from build123d import *

# Parameters (mm, degrees)
SKETCH_1_R                   = 26.5
EXTRUDE_2_DEPTH              = 5
SKETCH_3_R                   = 15
EXTRUDE_3_DEPTH              = 13
EXTRUDE_START                = 26.5
SKETCH_4_R                   = 15
EXTRUDE_4_DEPTH              = 26.5
HOLE_WIZARD_M4_1_D           = 3.3
HOLE_WIZARD_M4_1_CSINK_D     = 4.05
HOLE_WIZARD_M4_1_CSINK_ANGLE = 90
PATTERN_CIRCULAR_1_COUNT     = 6
SKETCH_7_R                   = 7.45
CUT_EXTRUDE_1_DEPTH          = 44.5
SKETCH_8_W                   = 5.01
SKETCH_8_H                   = 5
CUT_EXTRUDE_2_DEPTH          = 44.5


with BuildPart() as part:
    # 草图1 → 凸台-拉伸2 (new body)
    with BuildSketch(Plane(origin=(0, 0, 0), x_dir=(1, 0, 0), z_dir=(0, 1, 0))):
        with Locations(Location((0, 0, 0), (0, 0, 270))):
            Circle(SKETCH_1_R)
    extrude(amount=EXTRUDE_2_DEPTH)

    # 草图3 → 凸台-拉伸3 (add)
    with BuildSketch(Plane(origin=(0, 5, 0), x_dir=(1, 0, 0), z_dir=(0, 1, 0))):
        with Locations(Location((0, 0, 0), (0, 0, 90))):
            Circle(SKETCH_3_R)
    extrude(amount=EXTRUDE_3_DEPTH)

    # 草图4 → 凸台-拉伸4 (add)
    with BuildSketch(Plane.XZ.offset(EXTRUDE_START)):
        with Locations(Location((0, 0, 0), (0, 0, 270))):
            Circle(SKETCH_4_R)
    extrude(amount=-EXTRUDE_4_DEPTH)

    # M4 螺纹孔1 (through all)
    with Locations(Plane(origin=(22, 5, 0), x_dir=(0, 0, 1), z_dir=(0, 1, 0))):
        with Locations((0, 0)):
            hole_wizard_m4_1 = CounterSinkHole(HOLE_WIZARD_M4_1_D / 2, HOLE_WIZARD_M4_1_CSINK_D / 2, counter_sink_angle=HOLE_WIZARD_M4_1_CSINK_ANGLE)

    # 阵列(圆周)1: M4 螺纹孔1 ×6 about axis
    pattern_circular_1_axis = Axis((0, 0, 0), (0, 1, 0))
    for i in range(1, PATTERN_CIRCULAR_1_COUNT):
        add(hole_wizard_m4_1.rotate(pattern_circular_1_axis, i * 360 / PATTERN_CIRCULAR_1_COUNT), mode=Mode.SUBTRACT)

    # 草图7 → 切除-拉伸1 (cut)
    with BuildSketch(Plane(origin=(0, 18, 0), x_dir=(1, 0, 0), z_dir=(0, 1, 0))):
        with Locations(Location((0, 0, 0), (0, 0, 270))):
            Circle(SKETCH_7_R)
    extrude(amount=-CUT_EXTRUDE_1_DEPTH, mode=Mode.SUBTRACT)

    # 草图8 → 切除-拉伸2 (cut)
    with BuildSketch(Plane(origin=(0, 18, 0), x_dir=(1, 0, 0), z_dir=(0, 1, 0))):
        with Locations((0, -7.5)):
            Rectangle(SKETCH_8_W, SKETCH_8_H)
    extrude(amount=-CUT_EXTRUDE_2_DEPTH, mode=Mode.SUBTRACT)


solid = part.part
The model under review builds one solid part; all positions refer to its coordinate system, in mm. A direction names the side the tool comes from. Round coordinates to 2 decimals unless told otherwise and drop trailing zeros. Order: outer loops, then holes, each group sorted by start corner. A loop starts at its lowest first (then second) coordinate and runs counter-clockwise, first axis right, second up. Notation, with made-up numbers: (39, -22.75) -> (82, -22.75) arc R25 ccw to (82, -8.75) -> close; hole circle Ø7 at (-37, 39.25). An arc over 180 degrees is marked (long way). Use CSV: the item, a comma, the result in double quotes. Start each with the question number.
(1) Tool access review of faces 1 (the face through (0.66, -13.436, 14.985)), 2 (the face through (7, -26.5, -3)), 3 (the face through (0, -4, 10)): name each direction out of +Z, -Z, +X, -X, +Y, -Y from which nothing blocks a thin tool from reaching the whole face with its end or side.
(2) Consider section B-B on x = -4. Write out the cut boundary in (y, z), and give its area (3 significant figures).
(3) Consider section A-A on z = 0. Write out the cut boundary in (x, y) (3 decimals).
(4) Consider section D-D on y = 2.5. Write out the cut boundary in (x, z) (3 decimals).
(5) Insertion check: pin 1 (6 mm diameter, centred on x = 13.5, z = -17, fed in from +Y); pin 2 (12 mm diameter, centred on y = -8.5, z = -12, fed in from -X); pin 3 (6 mm diameter, centred on x = -14, y = -19, fed in from +Z); pin 4 (3 mm diameter, centred on x = 22, z = 0, fed in from -Y). Each pin has a flat end and moves straight along its axis. Give the tip position at first contact, or say it passes through.
(6) Wall thickness on probe 1 along X at (y, z) = (-9, 0); probe 2 along Y at (x, z) = (-1.5, 23); probe 3 along X at (y, z) = (12, 8) (3 decimals): over which ranges is each line inside the solid? List them lowest first. Write a range as from..to.
(7) Mouldability with a two-part tool opening along X and no side actions: class faces 4 (the face through (-0.66, 11.409, 14.985)), 5 (the face through (-7, 18, -3)), 6 (the face through (2.505, -4, 9)), 7 (the face through (-12, 2.28, -17.74)) as pulls with the +X half, pulls with the -X half, needs draft (parallel to the pull), parting line crosses it, or undercut.
(8) Consider section C-C on y = -7. Write out the cut boundary in (x, z) (3 decimals).
Responses:
1,face 1,"-Y"
1,face 2,"+Z, -Z, +X, -X, -Y"
1,face 3,"+Y, -Y"
2,outline,"(-26.5, -14.46) -> (0, -14.46) -> (0, -26.2) -> (5, -26.2) -> (5, -14.46) -> (18, -14.46) -> (18, -6.29) -> (-26.5, -6.29) -> close; (-26.5, 6.29) -> (18, 6.29) -> (18, 14.46) -> (5, 14.46) -> (5, 26.2) -> (0, 26.2) -> (0, 14.46) -> (-26.5, 14.46) -> close"
2,area,"845 mm²"
3,outline,"(-26.5, 0) -> (-23.65, 0) -> (-23.65, 4.625) -> (-24.025, 5) -> (-26.5, 5) -> close; (-20.35, 0) -> (-15, 0) -> (-15, -26.5) -> (-7.45, -26.5) -> (-7.45, 18) -> (-15, 18) -> (-15, 5) -> (-19.975, 5) -> (-20.35, 4.625) -> close; (7.45, -26.5) -> (15, -26.5) -> (15, 0) -> (20.35, 0) -> (20.35, 4.625) -> (19.975, 5) -> (15, 5) -> (15, 18) -> (7.45, 18) -> close; (23.65, 0) -> (26.5, 0) -> (26.5, 5) -> (24.025, 5) -> (23.65, 4.625) -> close"
4,outline,"circle Ø53 at (0, 0); hole circle Ø3.3 at (-22, 0); hole circle Ø3.3 at (-11, -19.053); hole circle Ø3.3 at (-11, 19.053); hole (-2.505, 7.016) arc R7.45 ccw (long way) to (2.505, 7.016) -> (2.505, 10) -> (-2.505, 10) -> close; hole circle Ø3.3 at (11, -19.053); hole circle Ø3.3 at (11, 19.053); hole circle Ø3.3 at (22, 0)"
5,pin 1,"y = 5"
5,pin 2,"x = -13.75"
5,pin 3,"z = 10.2"
5,pin 4,"through"
6,probe 1,"-15..-7.45, 7.45..15"
6,probe 2,"0..5"
6,probe 3,"-12.689..-2.505, 2.505..12.689"
7,face 4,"parting line crosses it"
7,face 5,"needs draft"
7,face 6,"undercut"
7,face 7,"undercut"
8,outline,"circle Ø30 at (0, 0); hole (-2.505, 7.016) arc R7.45 ccw (long way) to (2.505, 7.016) -> (2.505, 10) -> (-2.505, 10) -> close"
